Source: three-view drawing plus pictorial views. Frame: mm from the lowest corner of the part. A direction names the side the tool comes from. Give positions to 0.01 mm unless a question says otherwise; leave off trailing zeros. Write each loop counter-clockwise with the first axis right and the second up, starting at its lowest first coordinate (ties: lowest second). Pieces come first, ordered by that corner, then holes. Notation, with made-up numbers: (86, 55.5) -> (124, 55.5) arc R9 cw to (124, 71.5) -> close; hole circle Ø3 at (7.5, 89). An arc over 180 degrees is marked (long way). Write item = value, one per line.
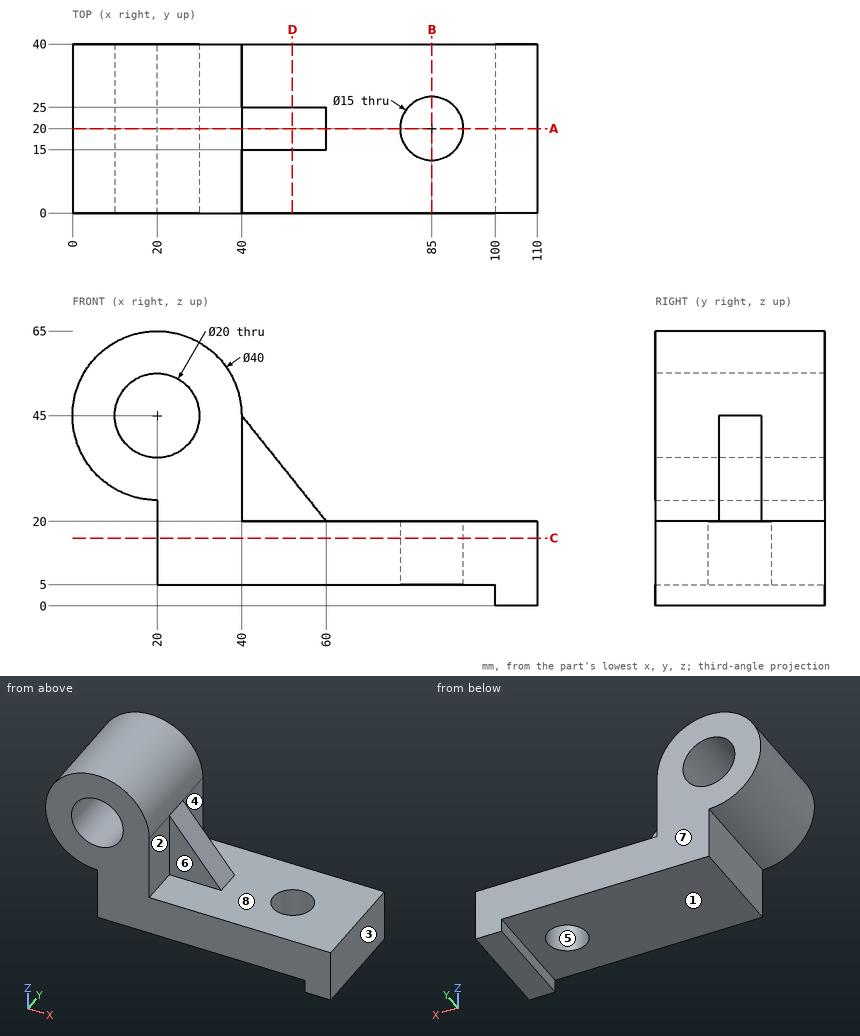
1) Access query for the marked faces 1, 2, 3 and 4. Directions: +Z, -Z, +X, -X, +Y, -Y. A direction counts if a zero-diameter tool reaches every point of the face in a straight line with its end or side. Return the directions, or none.
Computed:
face_1 = -Z, -X, +Y, -Y
face_2 = +Z, +X, -Y
face_3 = +Z, -Z, +X, +Y, -Y
face_4 = +Z, +X, +Y
2) Cut plane C-C (z = 16). Return the cut outline in (x, y), then the cut area to 3 significant figures.
Computed:
outline = (20, 0) -> (110, 0) -> (110, 40) -> (20, 40) -> close; hole circle Ø15 at (85, 20)
area = 3,420 mm²
3) Cut plane D-D (x = 52). Return the cut outline in (y, z), then the cut area to 3 significant figures.
Computed:
outline = (0, 5) -> (40, 5) -> (40, 20) -> (25, 20) -> (25, 30) -> (15, 30) -> (15, 20) -> (0, 20) -> close
area = 700 mm²
4) Cut plane B-B (x = 85). Return the cut outline in (y, z), then the cut area to 3 significant figures.
Computed:
outline = (0, 5) -> (12.5, 5) -> (12.5, 20) -> (0, 20) -> close; (27.5, 5) -> (40, 5) -> (40, 20) -> (27.5, 20) -> close
area = 375 mm²
5) Contact query for flat-ended pins moving along their axis: pin 1 (5 mm diameter, centred on y = 34, z = 13.5, fed in from -X); pin 2 (7.5 mm diameter, centred on y = 8, z = 28.5, fed in from +X); pin 3 (10 mm diameter, centred on x = 48, z = 31.5, fed in from +Y). Output: stop coordinate, or through.
Computed:
pin_1 = 20
pin_2 = 40
pin_3 = 25
6) Cut plane A-A (y = 20). Return the cut outline in (x, z).
Computed:
outline = (20, 5) -> (77.5, 5) -> (77.5, 20) -> (60, 20) -> (40, 45) arc R20 ccw (long way) to (20, 25) -> close; (92.5, 5) -> (100, 5) -> (100, 0) -> (110, 0) -> (110, 20) -> (92.5, 20) -> close; hole circle Ø20 at (20, 45)
7) Material intervals for L1, parallel to X at y = 14, z = 45; L2, parallel to X at y = 20, z = 12; L3, parallel to Y at x = 85, z = 15.5, sorted ascending.
Computed:
L1 = 0 to 10, 30 to 40
L2 = 20 to 77.5, 92.5 to 110
L3 = 0 to 12.5, 27.5 to 40
8) Draft query along Y for the marked faces 5, 6, 7 and 8. Return one class per face: pulls with the +Y half, pulls with the -Y half, needs draft (parallel to the pull), parting line crosses it, or undercut.
Computed:
face_5 = undercut
face_6 = pulls with the -Y half
face_7 = pulls with the +Y half
face_8 = needs draft
